Check sheet for the modelled part. Datum: model origin and axes. Units: mm. A direction names the side the tool comes from. Coordinates: 2 decimals unless noted, no trailing zeros. Order: outer loops, then holes, each group sorted by start corner. A loop starts at its lowest first (then second) coordinate and runs counter-clockwise, first axis right, second up.
Autodesk Inventor part; units mm, degrees
ref_plane "YZ Plane" through (0, 0, 0) normal (1, 0, 0) x (0, 1, 0)
ref_plane "XZ Plane" through (0, 0, 0) normal (0, 1, 0) x (-1, 0, 0)
ref_plane "XY Plane" through (0, 0, 0) normal (0, 0, 1) x (1, 0, 0)
sketch "Sketch1" plane through (0, 0, 0) normal (0, 0, 1) x (1, 0, 0)
  line L0 (-21.59, 0) -> (129.54, 0)
  line L1 (0, -7.62) -> (0, 45.72)
  line L2 (0, 0) -> (38.1, 38.1)
  line L3 (38.1, 38.1) -> (82.55, 38.1)
  line L4 (82.55, 38.1) -> (82.55, 31.75)
  line L5 (82.55, 31.75) -> (107.95, 31.75)
  line L6 (107.95, 31.75) -> (76.2, 0)
  line L7 (0, 0) -> (76.2, 0)
  dimension "d0" = 38.1
  dimension "d1" = 45
  dimension "d2" = 76.2
  dimension "d3" = 25.4
  dimension "d27" = 6.35
sketch "Sketch2" plane through (0, 0, 0) normal (0, 0, 1) x (1, 0, 0)
  point P0 (0, 0)
extrude "Extrusion1" add sketch "Sketch1" along normal blind 12.7
shell "Shell1" thickness 1.524 removed faces 1 at (38.1, 12.7, 12.7)
fillet "Fillet1" radius 3.175 6 edges at (38.7313, 36.576, 7.112) (81.026, 36.576, 7.112) (81.026, 30.226, 7.112) (104.2707, 30.226, 7.112) (75.5687, 1.524, 7.112) (3.6793, 1.524, 7.112)
sketch "Sketch3" plane through (11.3444, 1.524, 1.524) normal (0, 0, 1) x (1, 0, 0)
  line L0 (-11.3444, -1.524) -> (64.8556, -1.524)
  line L1 (-11.3444, -1.524) -> (7.7056, -1.524)
  line L2 (7.7056, -1.524) -> (7.7056, 6.35)
  circle A0 centre (7.7056, 6.35) radius 3.175
  line L3 (7.7056, 6.35) -> (25.6661, 24.3105) construction
  line L4 (-2.2451, 5.4201) -> (26.4569, 34.1221)
  circle A1 centre (25.6661, 24.3105) radius 3.175
  circle A2 centre (33.1056, 6.35) radius 3.175
  circle A3 centre (58.5056, 6.35) radius 3.175
  circle A4 centre (51.0661, 24.3105) radius 3.175
  circle A5 centre (76.4661, 24.3105) radius 3.175
  dimension "d32" = 19.05
  dimension "d33" = 7.874
  dimension "d35" = 25.4
  dimension "d41" = 25.4
  dimension "d42" = 25.4
  dimension "d46" = 6.35
  dimension "d47" = 25.4
  dimension "d48" = 25.4
extrude "Extrusion2" cut sketch "Sketch3" against normal through all
properties part number "Ch4 Part 1"
(1) Cross-section at A-A (x = 69.85). Enter the section's corners in (y, z).
Filled in:
outline: (0, 0) - (4.7, 0) - (4.7, 1.52) - (1.52, 1.52) - (1.52, 12.7) - (0, 12.7) - close; (11.05, 0) - (38.1, 0) - (38.1, 12.7) - (36.58, 12.7) - (36.58, 1.52) - (11.05, 1.52) - close
(2) Tool access check on faces 1 (the flat face through (23.249, 21.094, 7.034)), 2 (the flat face through (82.55, 35, 6)), 3 (the cylindrical face through (33.84, 25.97, 0.77)). Record the directions out of +Z, -Z, +X, -X, +Y, -Y that give a thin tool (end or side, any length) a straight path to the whole face; none if there is none.
Filled in:
face 1: +Z
face 2: +Z, -Z, +X, +Y
face 3: +Z, -Z
(3) Thickness scan on probe 1 along Y at (x, z) = (69.85, 0.8); probe 2 along Z at (x, y) = (68, 33); probe 3 along X at (y, z) = (17, 5). Record the ranges inside material, lowest first.
Filled in:
probe 1: y = 0 to 4.7, 11.05 to 38.1
probe 2: z = 0 to 1.52
probe 3: x = 17 to 19.16, 91.04 to 93.2
(4) Go/stop test with flat-tipped pins: P1, Ø3, axis at y = 13, z = 11.5, coming from the +X side; P2, Ø2, axis at x = 88, z = 6.5, coming from the -Y side; P3, Ø3.5, axis at x = 28, z = 6.5, coming from the +Y side. Record where each tip stops, or that it passes through.
Filled in:
P1: stops at x = 90.7
P2: stops at y = 10.8
P3: stops at y = 29.75
(5) Release check for a two-part mould opening along X. For faces 4 (the flat face through (54, 1, 12.7)), 5 (the flat face through (92.3, 16.1, 6.3)), 6 (the cylindrical face through (99.52, 28.31, 7.03)) record: +X half, -X half, draft (parallel to the pull), parting line (faces both ways), or undercut.
Filled in:
face 4: draft
face 5: +X half
face 6: undercut
(6) Cross-section at D-D (x = 49.5). Enter the section's corners in (y, z), and give its area (3 significant figures).
Filled in:
outline: (0, 0) - (38.1, 0) - (38.1, 12.7) - (36.58, 12.7) - (36.58, 1.52) - (1.52, 1.52) - (1.52, 12.7) - (0, 12.7) - close
area: 92.1 mm2
(7) Cross-section at C-C (y = 27). Enter the section's corners in (x, z).
Filled in:
outline: (27, 0) - (34.06, 0) - (34.06, 1.52) - (29.16, 1.52) - (29.16, 12.7) - (27, 12.7) - close; (39.96, 0) - (59.46, 0) - (59.46, 1.52) - (39.96, 1.52) - close; (65.36, 0) - (84.86, 0) - (84.86, 1.52) - (65.36, 1.52) - close; (90.76, 0) - (103.2, 0) - (103.2, 12.7) - (99.78, 12.7) - (99.78, 1.52) - (90.76, 1.52) - close
